```python
from build123d import *

# Parameters (mm, degrees)
SKETCH_1_W             = 80
SKETCH_1_H             = 70
EXTRUDE_1_DEPTH        = 70
SKETCH_2_W             = 64
SKETCH_2_H             = 32
CUT_EXTRUDE_1_DEPTH    = 60
SKETCH_3_R             = 4.5
CUT_EXTRUDE_5_DEPTH    = 100
SKETCH_6_R             = 5.5
CUT_EXTRUDE_7_DEPTH    = 30
SKETCH_5_R             = 20
CUT_EXTRUDE_8_DEPTH    = 87
SKETCH_7_R             = 23.5
CUT_EXTRUDE_9_DEPTH    = 14
FILLET_1_R             = 5
HOLE_WIZARD_M6_1_D     = 5
HOLE_WIZARD_M6_2_D     = 5
HOLE_WIZARD_M6_2_DEPTH = 10
HOLE_WIZARD_M6_2_TIP   = 1.502151548
HOLE_WIZARD_M6_3_D     = 5
HOLE_WIZARD_M6_3_DEPTH = 15
HOLE_WIZARD_M6_3_TIP   = 1.502151548


with BuildPart() as part:
    # 草图1 → 凸台-拉伸1 (new body)
    with BuildSketch(Plane.XY):
        Rectangle(SKETCH_1_W, SKETCH_1_H)
    extrude(amount=EXTRUDE_1_DEPTH)

    # 草图2 → 切除-拉伸1 (cut)
    with BuildSketch(Plane.XY.offset(70)):
        Rectangle(SKETCH_2_W, SKETCH_2_H)
    extrude(amount=-CUT_EXTRUDE_1_DEPTH, mode=Mode.SUBTRACT)

    # 草图3 → 切除-拉伸5 (cut)
    with BuildSketch(Plane.XY):
        with Locations((-33.5, 27.8)):
            Circle(SKETCH_3_R)
        with Locations((33.5, 27.8)):
            Circle(SKETCH_3_R)
        with Locations((33.5, -27.8)):
            Circle(SKETCH_3_R)
        with Locations((-33.5, -27.8)):
            Circle(SKETCH_3_R)
    extrude(amount=CUT_EXTRUDE_5_DEPTH, mode=Mode.SUBTRACT)

    # 草图6 → 切除-拉伸7 (cut)
    with BuildSketch(Plane(origin=(0, 0, 0), x_dir=(-1, 0, 0), z_dir=(0, 0, -1))):
        with Locations((-33.5, 27.8)):
            Circle(SKETCH_6_R)
        with Locations((33.5, 27.8)):
            Circle(SKETCH_6_R)
        with Locations((33.5, -27.8)):
            Circle(SKETCH_6_R)
        with Locations((-33.5, -27.8)):
            Circle(SKETCH_6_R)
    extrude(amount=-CUT_EXTRUDE_7_DEPTH, mode=Mode.SUBTRACT)

    # 草图5 → 切除-拉伸8 (cut)
    with BuildSketch(Plane(origin=(-5, 35, 0), x_dir=(0, 0, 1), z_dir=(0, -1, 0))):
        with Locations((35, -5)):
            Circle(SKETCH_5_R)
    extrude(amount=CUT_EXTRUDE_8_DEPTH, mode=Mode.SUBTRACT)

    # 草图7 → 切除-拉伸9 (cut)
    with BuildSketch(Plane.XZ.offset(-16)):
        with Locations((0, 35)):
            Circle(SKETCH_7_R)
    cut_extrude_9 = extrude(amount=-CUT_EXTRUDE_9_DEPTH, mode=Mode.SUBTRACT)

    # 镜向1: 切除-拉伸9 across plane
    add(cut_extrude_9.mirror(Plane(origin=(0, 0, 0), x_dir=(0, 0, 1), z_dir=(0, -1, 0))), mode=Mode.SUBTRACT)

    # 圆角1
    fillet_1_edges = [part.edges().sort_by_distance(p)[0] for p in [
        (32, 16, 40),
        (32, -16, 40),
        (-32, -16, 40),
        (-32, 16, 40),
    ]]
    fillet(fillet_1_edges, radius=FILLET_1_R)

    # M6 螺纹孔1 (through all)
    with Locations(Plane(origin=(-40, 7.5, 60), x_dir=(0, -1, 0), z_dir=(-1, 0, 0))):
        with Locations((0, 0), (15, 0)):
            Hole(HOLE_WIZARD_M6_1_D / 2)

    # M6 螺纹孔2
    with Locations(Plane(origin=(25, 35, 10), x_dir=(0, 0, 1), z_dir=(0, 1, 0))):
        with Locations((0, 0), (50, -50)):
            Hole(HOLE_WIZARD_M6_2_D / 2, depth=HOLE_WIZARD_M6_2_DEPTH)
            with Locations((0, 0, -(HOLE_WIZARD_M6_2_DEPTH + HOLE_WIZARD_M6_2_TIP / 2))):  # 118° drill point
                Cone(0, HOLE_WIZARD_M6_2_D / 2, HOLE_WIZARD_M6_2_TIP, mode=Mode.SUBTRACT)

    # M6 螺纹孔3
    with Locations(Plane(origin=(-25, -35, 60), x_dir=(0, 0, -1), z_dir=(0, -1, 0))):
        with Locations((0, 0), (0, 50), (50, 50), (50, 0)):
            Hole(HOLE_WIZARD_M6_3_D / 2, depth=HOLE_WIZARD_M6_3_DEPTH)
            with Locations((0, 0, -(HOLE_WIZARD_M6_3_DEPTH + HOLE_WIZARD_M6_3_TIP / 2))):  # 118° drill point
                Cone(0, HOLE_WIZARD_M6_3_D / 2, HOLE_WIZARD_M6_3_TIP, mode=Mode.SUBTRACT)


solid = part.part
```
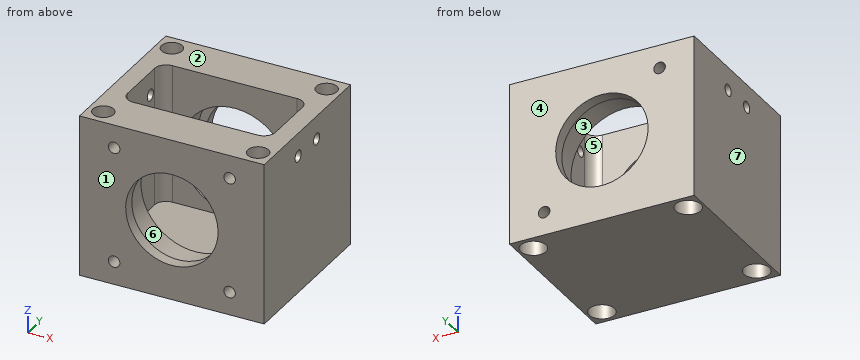
Model file for the job. Use its own axes, mm. Face numbers are marked on the shaded views. A direction names the side the tool comes from. Coordinates: 2 decimals unless noted, no trailing zeros. Loops run counter-clockwise (first coordinate to the right, second up) from the corner with the lowest first, then second, coordinate; pieces in that order, holes last. Notation, with made-up numbers: M 32.5,33.5 L 76.5,33.5 A14 ccw 76.5,48.5 Z; hole C -37.5,68.5 d3. An arc over 180 degrees is marked long. Use CSV: the item, a comma, the result in double quotes. Start each with the question number.
1. Flat gauge pin, fed straight in: pin 1 (5.5 mm diameter, centred on x = 34, y = 27, fed in from -Z). Where does the tip first touch, or does it go through?
2. Band-saw the part on C-C, the plane y = -7.5. List the corners of the cut face in (x, z), then the cut area to 3 significant figures.
3. Two-plate mould, pull along Y, no slides. Class the marked faces 1, 2, 3 and 4: pulls with the +Y half, pulls with the -Y half, needs draft (parallel to the pull), parting line crosses it, or undercut.
4. Tool access for the marked faces 5, 6 and 7: list every direction of +Z, -Z, +X, -X, +Y, -Y with a clear straight run to the whole face (end or side of a thin tool).
5. Band-saw the part on A-A, the plane z = 35. Give the number of separate pieces and of enclosed holes in the cut face, then the cut area to 3 significant figures.
6. Probe probe 1 along Y at (x, z) = (-33.5, 49.5); probe 2 along Z at (x, y) = (-25, -29.75); probe 3 along X at (y, z) = (2.5, 29). List the from-to ranges inside material, lowest first. Write a range as [from, to].
7. Band-saw the part on B-B, the plane x = 0. List the corners of the cut face in (y, z).
Entries:
1,pin 1,"passes through"
2,outline,"M -40,0 L 40,0 L 40,57.5 L 32,57.5 L 32,10 L -32,10 L -32,57.5 L -40,57.5 Z; M -40,62.5 L -32,62.5 L -32,70 L -40,70 Z; M 32,62.5 L 40,62.5 L 40,70 L 32,70 Z"
2,area,"1,680 mm2"
3,face 1,"pulls with the -Y half"
3,face 2,"needs draft"
3,face 3,"undercut"
3,face 4,"pulls with the +Y half"
4,face 5,"+Z"
4,face 6,"none"
4,face 7,"+Z, -Z, -X, +Y, -Y"
5,separate pieces,"2"
5,enclosed holes,"4"
5,area,"1,600 mm2"
6,probe 1,"y = [-35, -32.3], [-23.3, 23.3], [32.3, 35]"
6,probe 2,"z = [0, 7.5], [12.5, 57.5], [62.5, 70]"
6,probe 3,"x = [-40, -32], [32, 40]"
7,outline,"M -35,0 L 35,0 L 35,15 L 30,15 L 30,11.5 L 16,11.5 L 16,10 L -16,10 L -16,11.5 L -30,11.5 L -30,15 L -35,15 Z; M -35,55 L -30,55 L -30,58.5 L -16,58.5 L -16,70 L -35,70 Z; M 16,58.5 L 30,58.5 L 30,55 L 35,55 L 35,70 L 16,70 Z"
